Can you work these out from the model? Positions are in its coordinate system, mm. Face numbers are marked on the shaded views. A direction names the side the tool comes from. Coordinates: 2 decimals unless noted, no trailing zeros. Write each loop counter-clockwise with the first axis right and the second up, starting at its lowest first coordinate (ties: lowest second). Pieces come first, ordered by that corner, then holes. Notation, with made-up numbers: (27, 87.5) -> (38, 87.5) arc R23 ccw to (38, 105.5) -> close; hole circle Ø6 at (2.5, -31). An arc over 180 degrees is marked (long way). Answer as CSV lines item,"result". Start each with the question number.
```python
from build123d import *

# Parameters (mm, degrees)
SKETCH1_W           = 100
SKETCH1_H           = 100
BOSS_EXTRUDE1_DEPTH = 60
SKETCH2_W           = 60
SKETCH2_H           = 20
BOSS_EXTRUDE2_DEPTH = 50
SKETCH3_W           = 20
SKETCH3_H           = 60
BOSS_EXTRUDE3_DEPTH = 50
SKETCH4_R           = 15
CUT_EXTRUDE1_DEPTH  = 100
SKETCH5_R           = 15
CUT_EXTRUDE2_DEPTH  = 100


with BuildPart() as part:
    # Sketch1 → Boss-Extrude1 (new body)
    with BuildSketch(Plane.XY):
        Rectangle(SKETCH1_W, SKETCH1_H)
    extrude(amount=BOSS_EXTRUDE1_DEPTH)

    # Sketch2 → Boss-Extrude2 (add)
    with BuildSketch(Plane(origin=(50, 0, 0), x_dir=(0, 0, -1), z_dir=(1, 0, 0))):
        with Locations((-30, 40)):
            Rectangle(SKETCH2_W, SKETCH2_H)
        with Locations((-30, -40)):
            Rectangle(SKETCH2_W, SKETCH2_H)
    boss_extrude2 = extrude(amount=BOSS_EXTRUDE2_DEPTH)

    # Sketch3 → Boss-Extrude3 (add)
    with BuildSketch(Plane.XZ.offset(50)):
        with Locations((-40, 30)):
            Rectangle(SKETCH3_W, SKETCH3_H)
        with Locations((40, 30)):
            Rectangle(SKETCH3_W, SKETCH3_H)
    boss_extrude3 = extrude(amount=BOSS_EXTRUDE3_DEPTH)

    # Sketch4 → Cut-Extrude1 (cut)
    with BuildSketch(Plane.XZ.offset(50)):
        with Locations(Location((75, 30, 0), (0, 0, 270))):
            Circle(SKETCH4_R)
    cut_extrude1 = extrude(amount=-CUT_EXTRUDE1_DEPTH, mode=Mode.SUBTRACT)

    # Sketch5 → Cut-Extrude2 (cut)
    with BuildSketch(Plane(origin=(50, 0, 0), x_dir=(0, 0, -1), z_dir=(1, 0, 0))):
        with Locations((-30, -75)):
            Circle(SKETCH5_R)
    cut_extrude2 = extrude(amount=-CUT_EXTRUDE2_DEPTH, mode=Mode.SUBTRACT)

    # Mirror2: Boss-Extrude2, Cut-Extrude1 across plane
    add(boss_extrude2.mirror(Plane(origin=(0, 0, 0), x_dir=(0, 0, 1), z_dir=(1, 0, 0))))
    add(cut_extrude1.mirror(Plane(origin=(0, 0, 0), x_dir=(0, 0, 1), z_dir=(1, 0, 0))), mode=Mode.SUBTRACT)

    # Mirror3: Boss-Extrude3, Cut-Extrude2 across plane
    add(boss_extrude3.mirror(Plane.ZX))
    add(cut_extrude2.mirror(Plane.ZX), mode=Mode.SUBTRACT)


solid = part.part
```
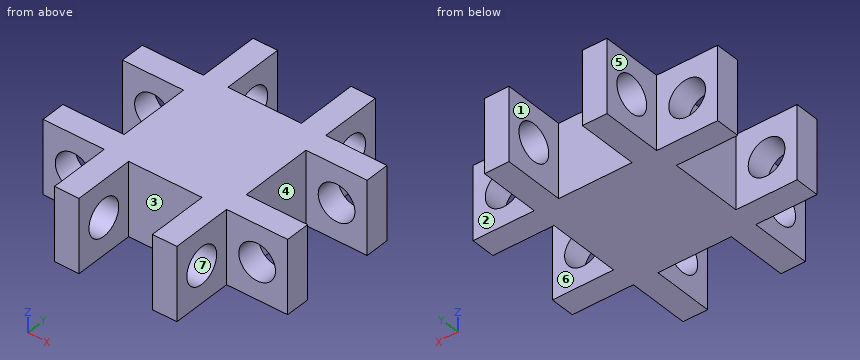
Q1. If we mould it in two halves opening along Z, with no side actions, what happens to the marked faces 6 and 7? For each: released by +Z, released by -Z, zero draft, split by the parting line, or undercut.
Q2. Imagine slicing it at C-C (z = 52.5). Write out the boundary of the cut face in (x, y), then the cut area to 3 significant figures.
Q3. Imagine slicing it at A-A (x = 66). Write out the boundary of the cut face in (y, z).
Q4. Imagine slicing it at B-B (y = -75). Write out the boundary of the cut face in (x, z).
Q5. Imagine slicing it at D-D (z = 18). State how many separate pieces and enclosed holes the cut face has, then the cut area to 3 significant figures.
Q6. For pin 1 (2 mm diameter, centred on x = -58, z = 27.5, fed in from -Y); pin 2 (15 mm diameter, centred on x = -86.5, z = 26, fed in from +Y); pin 3 (18 mm diameter, centred on y = -75, z = 30, fed in from -X); pin 4 (2 mm diameter, centred on y = 4, z = 48, fed in from -X), each with a flat end and sliding along its axis, tell me the tip position at first contact or that it passes through.
Q7. Which directions (+Z, -Z, +X, -X, +Y, -Y) give clear straight access to the entire face, cutting with the end or side of a thin tool? Please do the marked faces 1, 2, 3, 4 and 5.
Q8. I need wall thicknesses on L1, parallel to X at y = 39, z = 30; L2, parallel to Z at x = -75, y = -40. Which ranges of each line are inside material? Lowest first, please.
Entries:
1,face 6,"zero draft"
1,face 7,"undercut"
2,outline,"(-100, -50) -> (-50, -50) -> (-50, -100) -> (-30, -100) -> (-30, -50) -> (30, -50) -> (30, -100) -> (50, -100) -> (50, -50) -> (100, -50) -> (100, -30) -> (50, -30) -> (50, 30) -> (100, 30) -> (100, 50) -> (50, 50) -> (50, 100) -> (30, 100) -> (30, 50) -> (-30, 50) -> (-30, 100) -> (-50, 100) -> (-50, 50) -> (-100, 50) -> (-100, 30) -> (-50, 30) -> (-50, -30) -> (-100, -30) -> close"
2,area,"18,000 mm2"
3,outline,"(-50, 0) -> (-30, 0) -> (-30, 18) -> (-50, 18) -> close; (-50, 42) -> (-30, 42) -> (-30, 60) -> (-50, 60) -> close; (30, 0) -> (50, 0) -> (50, 18) -> (30, 18) -> close; (30, 42) -> (50, 42) -> (50, 60) -> (30, 60) -> close"
4,outline,"(-50, 0) -> (-30, 0) -> (-30, 15) -> (-50, 15) -> close; (-50, 45) -> (-30, 45) -> (-30, 60) -> (-50, 60) -> close; (30, 0) -> (50, 0) -> (50, 15) -> (30, 15) -> close; (30, 45) -> (50, 45) -> (50, 60) -> (30, 60) -> close"
5,separate pieces,"9"
5,enclosed holes,"0"
5,area,"15,100 mm2"
6,pin 1,"y = -50"
6,pin 2,"y = 50"
6,pin 3,"through"
6,pin 4,"x = -50"
7,face 1,"+Z, -Z, +Y"
7,face 2,"+Z, -Z, +X, +Y"
7,face 3,"+Z, -Z, -Y"
7,face 4,"+Z, -Z, +X"
7,face 5,"+Z, -Z, -X, +Y"
8,L1,"-100 to -90, -60 to 60, 90 to 100"
8,L2,"0 to 15, 45 to 60"
